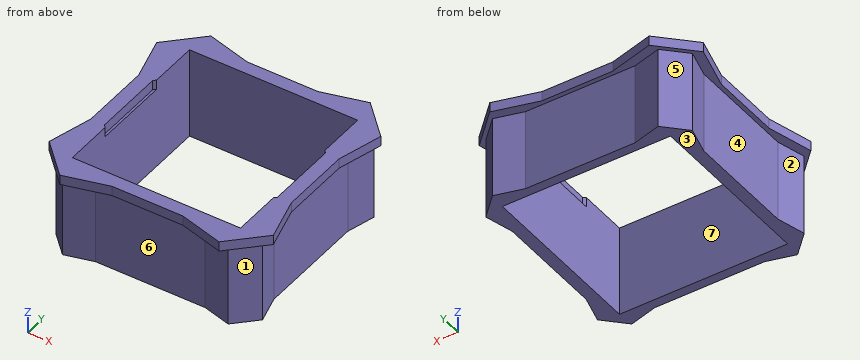
```python
from build123d import *

# Parameters (mm, degrees)
F5_DEPTH = 25.4
F6_DEPTH = 3.048
F7_W     = 52.44865641
F7_H     = 54.1748739779
F8_DEPTH = 88.646


with BuildPart() as f5:
    # F2 (on offset) → F5 (new body)
    with BuildSketch(Plane.XY.offset(50.292)):
        Polygon((-32.2327940663, -25.8321565638), (-25.8321565638, -32.2327940663), (-17.0887231349, -29.88999814), (-14.7459272086, -21.1465647111), (-21.1465647111, -14.7459272086), (-29.88999814, -17.0887231349), align=None)
        Polygon((-14.7459272086, -21.1465647111), (-17.0887231349, -29.88999814), (17.0887231349, -29.88999814), (14.7459272086, -21.1465647111), align=None)
        Polygon((-29.88999814, 17.0887231349), (-29.88999814, -17.0887231349), (-21.1465647111, -14.7459272086), (-21.1465647111, 14.7459272086), align=None)
        Polygon((14.7459272086, -21.1465647111), (17.0887231349, -29.88999814), (25.8321565638, -32.2327940663), (32.2327940663, -25.8321565638), (29.88999814, -17.0887231349), (21.1465647111, -14.7459272086), align=None)
        Polygon((-32.2327940663, 25.8321565638), (-29.88999814, 17.0887231349), (-21.1465647111, 14.7459272086), (-14.7459272086, 21.1465647111), (-17.0887231349, 29.88999814), (-25.8321565638, 32.2327940663), align=None)
        Polygon((21.1465647111, 14.7459272086), (21.1465647111, -14.7459272086), (29.88999814, -17.0887231349), (29.88999814, 17.0887231349), align=None)
        Polygon((-17.0887231349, 29.88999814), (-14.7459272086, 21.1465647111), (14.7459272086, 21.1465647111), (17.0887231349, 29.88999814), align=None)
        Polygon((14.7459272086, 21.1465647111), (21.1465647111, 14.7459272086), (29.88999814, 17.0887231349), (32.2327940663, 25.8321565638), (25.8321565638, 32.2327940663), (17.0887231349, 29.88999814), align=None)
    extrude(amount=F5_DEPTH)

    # F4 (on offset) → F6 (join)
    with BuildSketch(Plane.XY.offset(75.692)):
        Polygon((-24.8438008947, 34.9560788946), (-34.9560788946, 24.8438008947), (-31.2547282565, 11.0301722567), (-31.2547282565, -11.0301722567), (-34.9560788946, -24.8438008947), (-24.8438008947, -34.9560788946), (-11.0301722567, -31.2547282565), (11.0301722567, -31.2547282565), (24.8438008947, -34.9560788946), (34.9560788946, -24.8438008947), (31.2547282565, -11.0301722567), (31.2547282565, 11.0301722567), (34.9560788946, 24.8438008947), (24.8438008947, 34.9560788946), (11.0301722567, 31.2547282565), (-11.0301722567, 31.2547282565), align=None)
        Polygon((-26.953196153, 11.1643793959), (-11.1643793959, 26.953196153), (11.1643793959, 26.953196153), (26.953196153, 11.1643793959), (26.953196153, -11.1643793959), (11.1643793959, -26.953196153), (-11.1643793959, -26.953196153), (-26.953196153, -11.1643793959), align=None, mode=Mode.SUBTRACT)
    extrude(amount=F6_DEPTH)

    # F7 (on offset) → F8 (cut)
    with BuildSketch(Plane.XY.offset(50.292)):
        Rectangle(F7_W, F7_H)
    extrude(amount=F8_DEPTH, mode=Mode.SUBTRACT)


solid = f5.part
```
CAD build for the part. Positions are in the model's coordinates, mm. Face numbers are marked on the shaded views. A direction names the side the tool comes from. Coordinates: 2 decimals unless noted, no trailing zeros. Order: outer loops, then holes, each group sorted by start corner. A loop starts at its lowest first (then second) coordinate and runs counter-clockwise, first axis right, second up.
(1) Saw through at B-B, the plane x = -5.5. Write the cut outline in (y, z), and give its area (3 significant figures).
Solution:
outline: (-31.25, 75.69) - (-29.89, 75.69) - (-29.89, 50.29) - (-27.09, 50.29) - (-27.09, 78.74) - (-31.25, 78.74) - close; (27.09, 50.29) - (29.89, 50.29) - (29.89, 75.69) - (31.25, 75.69) - (31.25, 78.74) - (27.09, 78.74) - close
area: 168 mm2
(2) Pin check, flat tips, straight feed: pin 1 Ø3 at (y, z) = (14.5, 55.5) entering from +X; pin 2 Ø6 at (x, z) = (-26.5, 62.5) entering from +Y; pin 3 Ø4 at (y, z) = (2.5, 60) entering from -X; pin 4 Ø12 at (x, y) = (-2.5, -27) entering from -Z. Stop position of each tip, or through.
Solution:
pin 1: stops at x = 29.89
pin 2: stops at y = 32.23
pin 3: stops at x = -29.89
pin 4: stops at z = 50.29
(3) Mould opens along Y. For the marked faces 1, 2 and 3 say: released by +Y, released by -Y, zero draft, split by the parting line, or undercut.
Solution:
face 1: released by -Y
face 2: undercut
face 3: zero draft
(4) Saw through at C-C, the plane z = 52.5. Write the cut outline in (x, y), and give its area (3 significant figures).
Solution:
outline: (-32.23, -25.83) - (-25.83, -32.23) - (-17.09, -29.89) - (17.09, -29.89) - (25.83, -32.23) - (32.23, -25.83) - (29.89, -17.09) - (29.89, 17.09) - (32.23, 25.83) - (25.83, 32.23) - (17.09, 29.89) - (-17.09, 29.89) - (-25.83, 32.23) - (-32.23, 25.83) - (-29.89, 17.09) - (-29.89, -17.09) - close; hole (-26.22, -27.09) - (26.22, -27.09) - (26.22, 27.09) - (-26.22, 27.09) - close
area: 830 mm2
(5) Which spindle directions (+Z, -Z, +X, -X, +Y, -Y) get a long thin tool onto all of the face, cutting with end or side? Do the marked faces 4, 5, 6 and 7. Say none if no direction does.
Solution:
face 4: -Z, -X
face 5: -Z, -X, +Y
face 6: -Z, -Y
face 7: +Z, -Z
(6) Drill centre lines: L1, parallel to X at y = -6.5, z = 71; L2, parallel to Y at x = -8.5, z = 56.5; L3, parallel to Y at x = 24, z = 74.5. Where is each one in solid material? Low to high.
Solution:
L1: x = -29.89 to -26.22, 26.22 to 29.89
L2: y = -29.89 to -27.09, 27.09 to 29.89
L3: y = -31.74 to -27.09, 27.09 to 31.74
(7) Saw through at A-A, the plane y = -3. Write the cut outline in (x, z), and give its area (3 significant figures).
Solution:
outline: (-31.25, 75.69) - (-29.89, 75.69) - (-29.89, 50.29) - (-26.22, 50.29) - (-26.22, 75.69) - (-26.95, 75.69) - (-26.95, 78.74) - (-31.25, 78.74) - close; (26.22, 50.29) - (29.89, 50.29) - (29.89, 75.69) - (31.25, 75.69) - (31.25, 78.74) - (26.95, 78.74) - (26.95, 75.69) - (26.22, 75.69) - close
area: 212 mm2
(8) Saw through at D-D, the plane x = -28.5. Write the cut outline in (y, z), and give its area (3 significant figures).
Solution:
outline: (-31.3, 75.69) - (-29.56, 75.69) - (-29.56, 50.29) - (29.56, 50.29) - (29.56, 75.69) - (31.3, 75.69) - (31.3, 78.74) - (-31.3, 78.74) - close
area: 1,690 mm2
